The drawing under review shows one solid part. Ordinate dimensions are in mm from its lowest x, y, z. A direction names the side the tool comes from. Give positions to 0.01 mm unless a question says otherwise; leave off trailing zeros. Loops run counter-clockwise (first coordinate to the right, second up) from the corner with the lowest first, then second, coordinate; pieces in that order, holes last. Notation, with made-up numbers: (18.25, 66) -> (75.25, 66) arc R13 ccw to (75.25, 86) -> close; hole circle Ø7 at (22, 87.5). An arc over 180 degrees is marked (long way). Answer in a Markdown table with one row per item. Add a question column.
(1) For line 1 (Z direction, x = 19, y = 5); line 2 (X direction, y = 19, z = 4); line 3 (X direction, y = 18, z = 5), list the stretches that pass through material, from the lowest coordinate up.
(2) Consider section A-A on x = 6.25. Write out the cut boundary in (y, z), then the cut area to 3 significant figures.
(3) Consider section C-C on x = 1.75. Write out the cut boundary in (y, z).
(4) Consider section B-B on y = 18.75. Write out the cut boundary in (x, z).
(5) For pin 1 (0.6 mm diameter, centred on y = 17, z = 6, fed in from +X); pin 2 (10 mm diameter, centred on x = 6, y = 11, fed in from +Z); pin 3 (2 mm diameter, centred on y = 17, z = 5, fed in from -X), all flat-tipped, find the tip position at first contact; note any pin that passes through.
(6) For the marked faces 1 and 2, list the 3-axis set-ups (+Z, -Z, +X, -X, +Y, -Y) from which the entire face can be reached by the end or side of a thin tool; tool diameter is ignored.
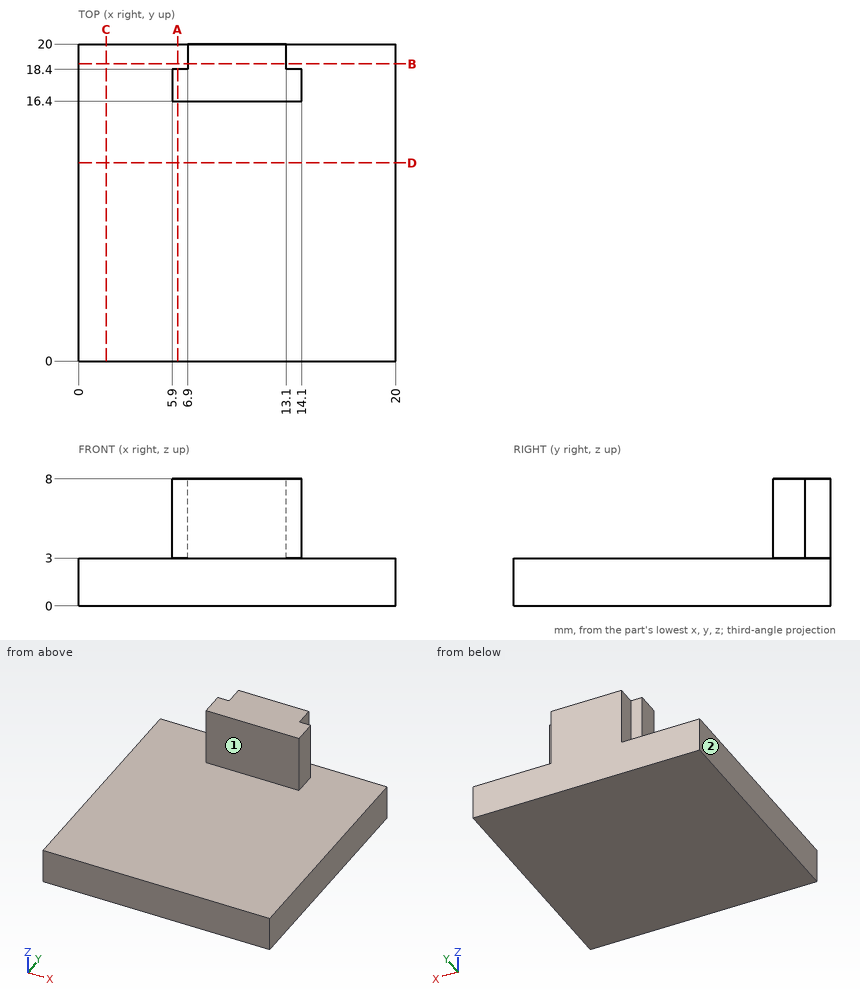
Values follow:
| question | item | result |
|---|---|---|
| 1 | line 1 | 0 to 3 |
| 1 | line 2 | 6.9 to 13.1 |
| 1 | line 3 | 5.9 to 14.1 |
| 2 | outline | (0, 0) -> (20, 0) -> (20, 3) -> (18.4, 3) -> (18.4, 8) -> (16.4, 8) -> (16.4, 3) -> (0, 3) -> close |
| 2 | area | 70.0 mm2 |
| 3 | outline | (0, 0) -> (20, 0) -> (20, 3) -> (0, 3) -> close |
| 4 | outline | (0, 0) -> (20, 0) -> (20, 3) -> (13.1, 3) -> (13.1, 8) -> (6.9, 8) -> (6.9, 3) -> (0, 3) -> close |
| 5 | pin 1 | x = 14.1 |
| 5 | pin 2 | z = 3 |
| 5 | pin 3 | x = 5.9 |
| 6 | face 1 | +Z, +X, -X, -Y |
| 6 | face 2 | +Z, -Z, -X, +Y, -Y |
